Verification items for the finished model (mm, model axes). Face numbers are marked on the shaded views. A direction names the side the tool comes from. Coordinates: 2 decimals unless noted, no trailing zeros. Write each loop counter-clockwise with the first axis right and the second up, starting at its lowest first coordinate (ties: lowest second). Pieces come first, ordered by that corner, then holes. Notation, with made-up numbers: (19, 55) -> (51, 55) arc R14 cw to (51, 78) -> close; hole circle Ø3 at (9.5, 69). An arc over 180 degrees is marked (long way). Use a Markdown table: item, result. Add a question column.
from build123d import *

# Parameters (mm, degrees)
BOSS_EXTRU_1_DEPTH = 50
NERVURE1_START     = -5
NERVURE1_DEPTH     = 5
D_GAGEMENT_51_D    = 11.0744


# Read off the part's stored shape, not the designer's step: Nervure1
with BuildPart() as part:
    # Esquisse1 → Boss.-Extru.1 (new, symmetric)
    with BuildSketch(Plane.XY):
        Polygon((-67.326566733, 0), (67.742162824, 0), (67.742162824, 8.623618887), (-52.78070355, 8.623618887), (-52.78070355, 68.053859892), (-67.326566733, 68.053859892), align=None)
    extrude(amount=BOSS_EXTRU_1_DEPTH, both=True)

    # Nervure1 outline → Nervure1 (add)
    with BuildSketch(Plane.XY.offset(30).offset(NERVURE1_START)):
        with BuildLine():
            Line((19.279550654, 8.623618887), (-6.210494082, 34.113663623))
            ThreePointArc((-6.210494082, 34.113663623), (-15.230796531, 30.377332012), (-24.251098981, 34.113663623))
            Line((-24.251098981, 34.113663623), (-52.78070355, 62.643268192))
            Line((-52.78070355, 62.643268192), (-52.78070355, 8.623618887))
            Line((-52.78070355, 8.623618887), (19.279550654, 8.623618887))
        make_face()
    nervure1 = extrude(amount=NERVURE1_DEPTH)

    # Symétrie1: Nervure1 across plane
    add(nervure1.mirror(Plane.XY))

    # Dégagement #51 (through all)
    with Locations(Plane(origin=(0, 0, -30), x_dir=(-1, 0, 0), z_dir=(0, 0, -1))):
        with Locations((27.78070355, 18.623618887)):
            Hole(D_GAGEMENT_51_D / 2)


solid = part.part
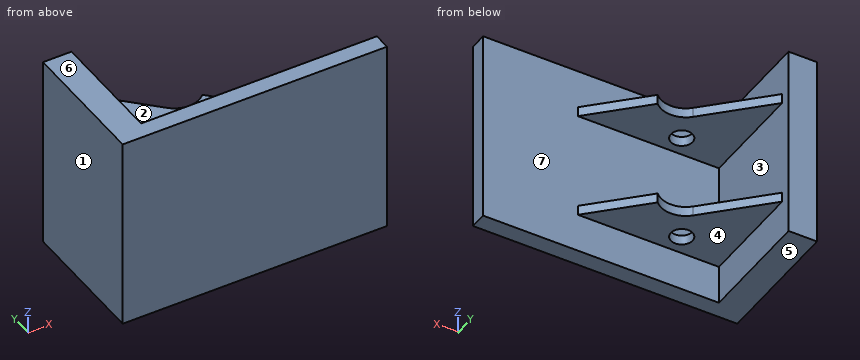
1) Cross-section at A-A on y = 15. Record the boundary of the cut face in (x, z), then the cut area to 3 significant figures.
2) Cross-section at C-C on y = 59. Record the boundary of the cut face in (x, z), then the cut area to 3 significant figures.
3) Gauge pin test, flat ends, axial feed: pin 1 (18 mm diameter, centred on y = 39.5, z = 14, fed in from +X); pin 2 (9 mm diameter, centred on x = -27.78, y = 18.62, fed in from +Z); pin 3 (1 mm diameter, centred on x = 23, z = 37.5, fed in from +Y); pin 4 (12 mm diameter, centred on x = -43, z = -35, fed in from +Y). Record the tip position at first contact, or that the pin passes through.
4) Release check for a two-part mould opening along Z. For the marked faces 5, 6 and 7 record: released by +Z, released by -Z, zero draft, split by the parting line, or undercut.
5) Cross-section at B-B on x = -26. Record the boundary of the cut face in (y, z), then the cut area to 3 significant figures.
6) Cross-section at D-D on x = 15. Record the boundary of the cut face in (y, z).
7) Set-up check for the marked faces 1, 2, 3 and 4: record each of +Z, -Z, +X, -X, +Y, -Y from which the full face is reachable in a straight line by a thin tool's end or side.
8) Thickness scan on L1, parallel to Z at x = -31.5, y = 23; L2, parallel to Y at x = 28.5, z = -41.5; L3, parallel to X at y = 55, z = 34.5. Record the ranges inside material, lowest first.
Returned:
| question | item | result |
|---|---|---|
| 1 | outline | (-67.33, -50) -> (-52.78, -50) -> (-52.78, -30) -> (-31.97, -30) -> (-31.97, -25) -> (-52.78, -25) -> (-52.78, 25) -> (-31.97, 25) -> (-31.97, 30) -> (-52.78, 30) -> (-52.78, 50) -> (-67.33, 50) -> close; (-23.59, -30) -> (12.9, -30) -> (12.9, -25) -> (-23.59, -25) -> close; (-23.59, 25) -> (12.9, 25) -> (12.9, 30) -> (-23.59, 30) -> close |
| 1 | area | 2,030 mm² |
| 2 | outline | (-67.33, -50) -> (-52.78, -50) -> (-52.78, -30) -> (-49.14, -30) -> (-49.14, -25) -> (-52.78, -25) -> (-52.78, 25) -> (-49.14, 25) -> (-49.14, 30) -> (-52.78, 30) -> (-52.78, 50) -> (-67.33, 50) -> close |
| 2 | area | 1,490 mm² |
| 3 | pin 1 | stops at x = -52.78 |
| 3 | pin 2 | passes through |
| 3 | pin 3 | stops at y = 8.62 |
| 3 | pin 4 | stops at y = 56.18 |
| 4 | face 5 | released by -Z |
| 4 | face 6 | released by +Z |
| 4 | face 7 | undercut |
| 5 | outline | (0, -50) -> (8.62, -50) -> (8.62, -30) -> (13.38, -30) -> (13.38, -25) -> (8.62, -25) -> (8.62, 25) -> (13.38, 25) -> (13.38, 30) -> (8.62, 30) -> (8.62, 50) -> (0, 50) -> close; (23.87, -30) -> (35.86, -30) -> (35.86, -25) -> (23.87, -25) -> close; (23.87, 25) -> (35.86, 25) -> (35.86, 30) -> (23.87, 30) -> close |
| 5 | area | 1,030 mm² |
| 6 | outline | (0, -50) -> (8.62, -50) -> (8.62, -30) -> (12.9, -30) -> (12.9, -25) -> (8.62, -25) -> (8.62, 25) -> (12.9, 25) -> (12.9, 30) -> (8.62, 30) -> (8.62, 50) -> (0, 50) -> close |
| 7 | face 1 | +Z, -Z, -X, +Y, -Y |
| 7 | face 2 | +Z, +X, +Y |
| 7 | face 3 | +X, +Y |
| 7 | face 4 | -Z, +X, +Y |
| 8 | L1 | z = -30 to -25, 25 to 30 |
| 8 | L2 | y = 0 to 8.62 |
| 8 | L3 | x = -67.33 to -52.78 |
